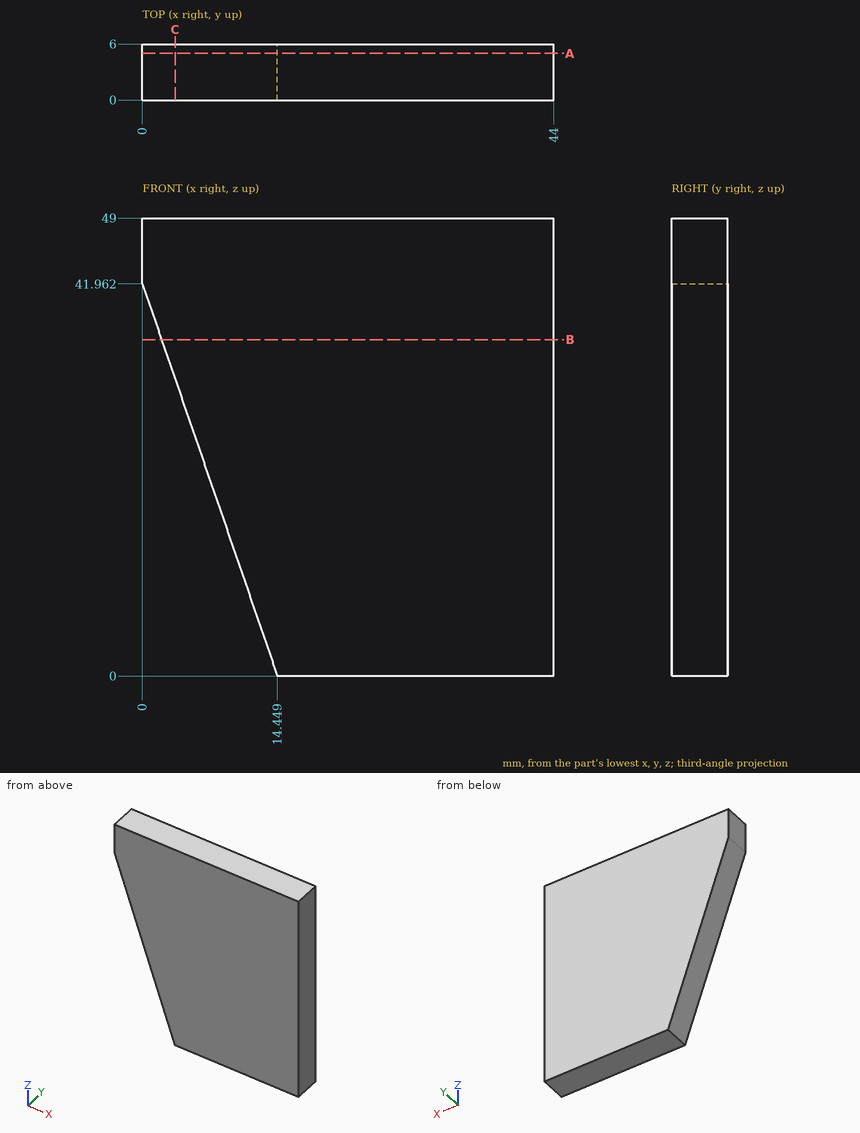
Could you check a few things on this drawing? It's one solid part, dimensions in mm from its lowest x, y, z. Round coordinates to 2 decimals unless told otherwise and drop trailing zeros. Order: outer loops, then holes, each group sorted by start corner. A loop starts at its lowest first (then second) coordinate and runs counter-clockwise, first axis right, second up. Notation, with made-up numbers: M 52,7 L 94,7 A26 ccw 94,37 Z; hole C 24.25,41 d1. An arc over 180 degrees is marked long. Return JSON: item names as keys, results as strings. Group by question number.
1. I'm going to push a flat-ended pin straight in: pin 1 Ø1.5 at (y, z) = (2.5, 25.5) entering from -X. Where does the tip first touch, or does it pass through?
2. Please list where these lines run through material, in increasing order: probe 1 along X at (y, z) = (5.55, 28); probe 2 along X at (y, z) = (3.5, 17) (1 decimal).
3. If we section it at A-A on y = 5: List the corners of the cut face in (x, z) for me.
4. If we section it at B-B on z = 36: List the corners of the cut face in (x, y) for me, then the cut area to 3 significant figures.
5. If we section it at C-C on x = 3.5: List the corners of the cut face in (y, z) for me.
Reply:
{
 "1": {"pin 1": "x = 5.41"},
 "2": {"probe 1": "4.81 to 44", "probe 2": "8.6 to 44"},
 "3": {"outline": "M 0,41.96 L 14.45,0 L 44,0 L 44,49 L 0,49 Z"},
 "4": {"outline": "M 2.05,0 L 44,0 L 44,6 L 2.05,6 Z", "area": "252 mm^2"},
 "5": {"outline": "M 0,31.8 L 6,31.8 L 6,49 L 0,49 Z"}
}
